from build123d import *

# Parameters (mm, degrees)
F0_R     = 41.275
F0_R_2   = 28.575
F1_DEPTH = 6.35
F2_R     = 34.925
F3_DEPTH = 3.175
F5_D     = 4.0386
F5_DEPTH = 6.35
F5_TIP   = 1.213317848


with BuildPart() as f1:
    # F0 (on Front) → F1 (new body)
    with BuildSketch(Plane.XZ):
        Circle(F0_R)
        Circle(F0_R_2, mode=Mode.SUBTRACT)
    extrude(amount=F1_DEPTH)

    # F2 (on face) → F3 (cut)
    with BuildSketch(Plane.XZ.offset(6.35)):
        Circle(F2_R)
    extrude(amount=-F3_DEPTH, mode=Mode.SUBTRACT)

    # F5
    with Locations(Plane.XZ.offset(6.35)):
        with Locations((-32.0266075904, 20.6375), (32.0266075904, 20.6375), (32.0266075904, -20.6375), (-32.0266075904, -20.6375)):
            Hole(F5_D / 2, depth=F5_DEPTH)
            with Locations((0, 0, -(F5_DEPTH + F5_TIP / 2))):  # 118° drill point
                Cone(0, F5_D / 2, F5_TIP, mode=Mode.SUBTRACT)


solid = f1.part
Geometry: final body of the model. Coordinates: model frame, mm. A direction names the side the tool comes from. Give positions to 0.01 mm unless a question says otherwise; leave off trailing zeros. Write each loop counter-clockwise with the first axis right and the second up, starting at its lowest first coordinate (ties: lowest second). Pieces come first, ordered by that corner, then holes.
(1) Cut plane B-B, the plane z = 0. Return loops of the section in (x, y) (3 decimals).
(2) Access query for faces 1 (the flat face through (-29, -3.175, 0)), 2 (the flat face through (-10, 0, -27)). Directions: +Z, -Z, +X, -X, +Y, -Y. A direction counts if a zero-diameter tool reaches every point of the face in a straight line with its end or side. Return the directions, or none.
(3) Cut plane C-C, the plane y = -1.5. Give the number of separate pieces and of enclosed holes in the cut face, then the cut area to 3 significant figures.
(4) Ray query, line 1 (Z direction, x = 0, y = -3.8) (3 decimals); line 2 (X direction, y = -4, z = 19); line 3 (Y direction, x = -34.5, z = 1) (3 decimals). Return the intervals inside material, ascending.
(5) Cut plane A-A, the plane x = 0. Return loops of the section in (y, z) (3 decimals), then the cut area to 3 significant figures.
(6) Mould query, pull axis Z, two halves, no side actions, for faces 3 (the cylindrical face through (33.515, -3.131, 22.002)), 4 (the cylindrical face through (-27.715, -4.785, -21.251)), 5 (the flat face through (-34, -6.35, 9)), 6 (the cylindrical face through (-8.948, -3.131, -40.293)). Classes: released by +Z, released by -Z, zero draft, split by the parting line, or undercut.
(7) First-contact query: P1, Ø2, axis at y = -1, z = -3, coming from the -X side; P2, Ø2.5, axis at x = 32.03, z = -20.64, coming from the +Y side. Flat tips, straight axial feed; report the tip coordinate or a pass-through.
Values follow:
1. outline: (-41.275, -6.35) - (-34.925, -6.35) - (-34.925, -3.175) - (-28.575, -3.175) - (-28.575, 0) - (-41.275, 0) - close; (28.575, -3.175) - (34.925, -3.175) - (34.925, -6.35) - (41.275, -6.35) - (41.275, 0) - (28.575, 0) - close
2. face 1: -Y
2. face 2: +Z, -Z, +X, -X, +Y
3. separate pieces: 1
3. enclosed holes: 5
3. area: 2,740 mm2
4. line 1: z = -41.275 to -34.925, 34.925 to 41.275
4. line 2: x = -36.64 to -33.21, -30.85 to -29.3, 29.3 to 30.85, 33.21 to 36.64
4. line 3: y = -3.175 to 0
5. outline: (-6.35, -41.275) - (0, -41.275) - (0, -28.575) - (-3.175, -28.575) - (-3.175, -34.925) - (-6.35, -34.925) - close; (-6.35, 34.925) - (-3.175, 34.925) - (-3.175, 28.575) - (0, 28.575) - (0, 41.275) - (-6.35, 41.275) - close
5. area: 121 mm2
6. face 3: undercut
6. face 4: undercut
6. face 5: zero draft
6. face 6: split by the parting line
7. P1: stops at x = -41.23
7. P2: passes through
